The drawing under review shows one solid part. Ordinate dimensions are in mm from its lowest x, y, z. Round coordinates to 2 decimals unless told otherwise and drop trailing zeros. Write each loop counter-clockwise with the first axis right and the second up, starting at its lowest first coordinate (ties: lowest second). Pieces come first, ordered by that corner, then holes.
Item 1: Clearance check with flat-ended pins moving along their axes: pin 1 Ø2 at (y, z) = (85.5, 114.5) entering from +X; pin 2 Ø2 at (x, z) = (97.5, 148) entering from +Y; pin 3 Ø5 at (x, z) = (150, 290.5) entering from -Y. State where each tip first meets the part, or that it passes through.
Item 2: Add section A-A (z = 214.5). Give the boundary of the cut face in (x, y) (1 decimal).
Item 3: Add section C-C (x = 81). Give the boundary of the cut face in (y, z) (1 decimal).
Item 4: Add section D-D (z = 151). Give the boundary of the cut face in (x, y) (1 decimal).
Item 5: To check wall thickness, follow L1, parallel to Z at x = 240, y = 96 (1 decimal); L2, parallel to Y at x = 79, z = 229.5; L3, parallel to X at y = 91.5, z = 99. State the ranges of each line that lie inside material, in increasing order.
Item 6: Add section B-B (y = 109). Give the boundary of the cut face in (x, z) (1 decimal), plus the area to 3 significant figures.
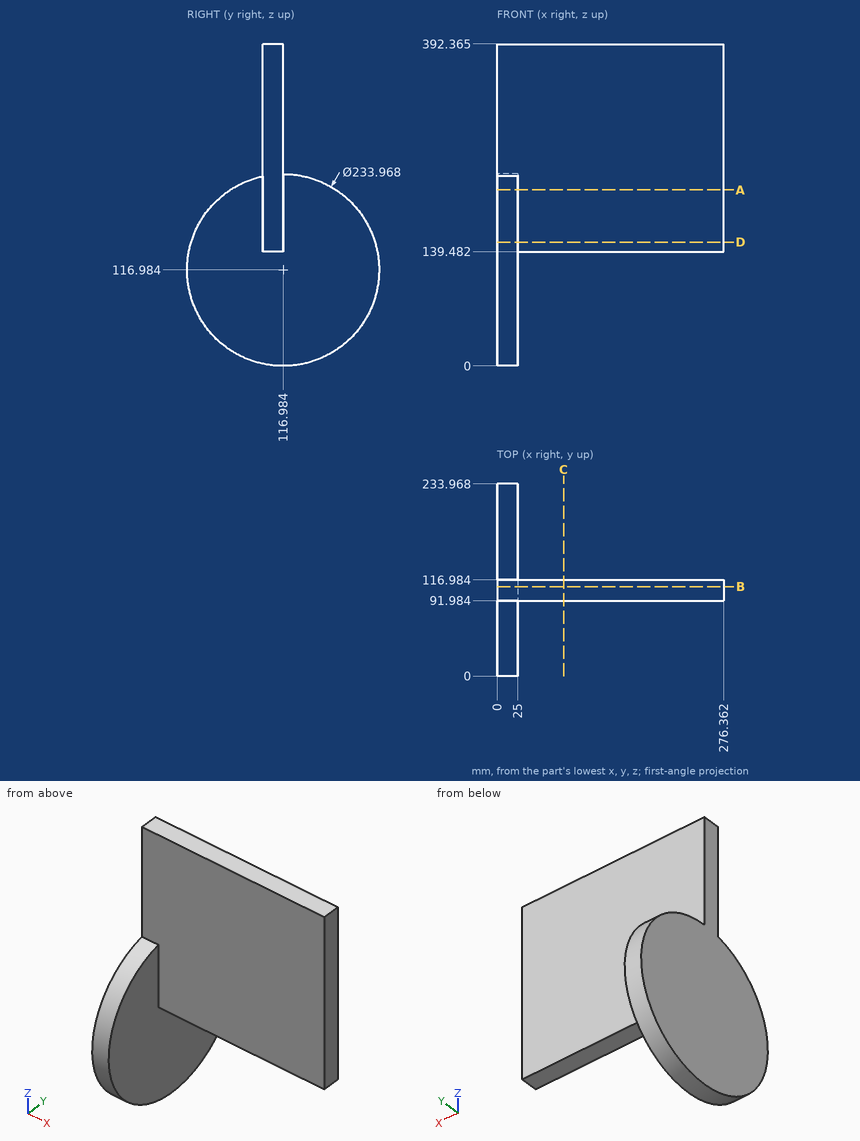
Numbers:
1. pin 1: stops at x = 25
1. pin 2: stops at y = 116.98
1. pin 3: stops at y = 91.98
2. outline: (0, 52.4) - (25, 52.4) - (25, 92) - (276.4, 92) - (276.4, 117) - (25, 117) - (25, 181.6) - (0, 181.6) - close
3. outline: (92, 139.5) - (117, 139.5) - (117, 392.4) - (92, 392.4) - close
4. outline: (0, 5.1) - (25, 5.1) - (25, 92) - (276.4, 92) - (276.4, 117) - (25, 117) - (25, 228.9) - (0, 228.9) - close
5. L1: z = 139.5 to 392.4
5. L2: y = 91.98 to 116.98
5. L3: x = 0 to 25
6. outline: (0, 0.3) - (25, 0.3) - (25, 139.5) - (276.4, 139.5) - (276.4, 392.4) - (0, 392.4) - close
6. area: 73,400 mm2
